Work out the finished part from the listing and answer in its coordinate system (mm). A direction names the side the tool comes from. Round coordinates to 2 decimals unless told otherwise and drop trailing zeros. Order: outer loops, then holes, each group sorted by start corner. A loop starts at its lowest first (then second) coordinate and runs counter-clockwise, first axis right, second up. Notation, with made-up numbers: (66.5, -4.75) -> (100.5, -4.75) arc R29 cw to (100.5, 27.25) -> close; hole circle Ø6 at (71.25, -13.5). An arc over 180 degrees is marked (long way). Use one line per item in the form item = value.
```python
from build123d import *

# Parameters (mm, degrees)
F0_W     = 38.1
F0_H     = 25.4
F1_DEPTH = 12.7
F3_START = 6.35
F2_W     = 12.7
F2_H     = 12.7
F3_DEPTH = 19.05
F4_W     = 12.7
F4_H     = 6.35
F5_DEPTH = 25.4


with BuildPart() as f1:
    # F0 (on Front) → F1 (new body, symmetric)
    with BuildSketch(Plane.XZ):
        with Locations((19.05, 12.7)):
            Rectangle(F0_W, F0_H)
    extrude(amount=F1_DEPTH, both=True)

    # F2 (on Front) → F3 (cut)
    with BuildSketch(Plane.XZ.offset(F3_START)):
        with Locations((31.75, 19.05)):
            Rectangle(F2_W, F2_H)
    extrude(amount=F3_DEPTH, mode=Mode.SUBTRACT)

    # F4 (on Top) → F5 (cut)
    with BuildSketch(Plane.XY):
        with Locations((6.35, 9.525)):
            Rectangle(F4_W, F4_H)
    extrude(amount=-F5_DEPTH, mode=Mode.SUBTRACT)


solid = f1.part
```
Item 1: Flat-ended cylindrical pins translate along their axes: P1, Ø4, axis at y = 7, z = 21, coming from the -X side; P2, Ø3, axis at y = -9.5, z = 22, coming from the +X side; P3, Ø1.9, axis at x = 35, y = -9.5, coming from the +Z side. Find the tip coordinate at first contact, or state that the pin passes through.
Findings:
P1 = 0
P2 = 25.4
P3 = 12.7
Item 2: The part is cut by section B-B, the plane x = 32.5. Give the vertices of the cut face in (y, z).
Findings:
outline = (-12.7, 0) -> (12.7, 0) -> (12.7, 25.4) -> (-6.35, 25.4) -> (-6.35, 12.7) -> (-12.7, 12.7) -> close
Item 3: For faces 1 (the flat face through (19, 0, 0)), 2 (the flat face through (32, -6.35, 19)), determine the directions among +Z, -Z, +X, -X, +Y, -Y from which every point of the face is accessible in a straight line to the end or side of a thin tool.
Findings:
face_1 = -Z, +X, -X, +Y, -Y
face_2 = +Z, +X, -Y
Item 4: The part is cut by section A-A, the plane y = -8.75. Give the vertices of the cut face in (x, z).
Findings:
outline = (0, 0) -> (38.1, 0) -> (38.1, 12.7) -> (25.4, 12.7) -> (25.4, 25.4) -> (0, 25.4) -> close
Item 5: Consider line 1 along X through (y, z) = (-7.75, 22.5). Determine where the line is inside the solid, lowest interval first.
Findings:
line_1 = 0 to 25.4
